Part print with two shaded views. Sizes in mm from the minimum x, y, z corner. A direction names the side the tool comes from. Give positions to 0.01 mm unless a question says otherwise; leave off trailing zeros. Loops run counter-clockwise (first coordinate to the right, second up) from the corner with the lowest first, then second, coordinate; pieces in that order, holes last. Notation, with made-up numbers: M 30.5,65 L 81.5,65 A29 ccw 81.5,87 Z; hole C 84.5,68.25 d1. An arc over 180 degrees is marked long. Answer in a Markdown table with one row per item.
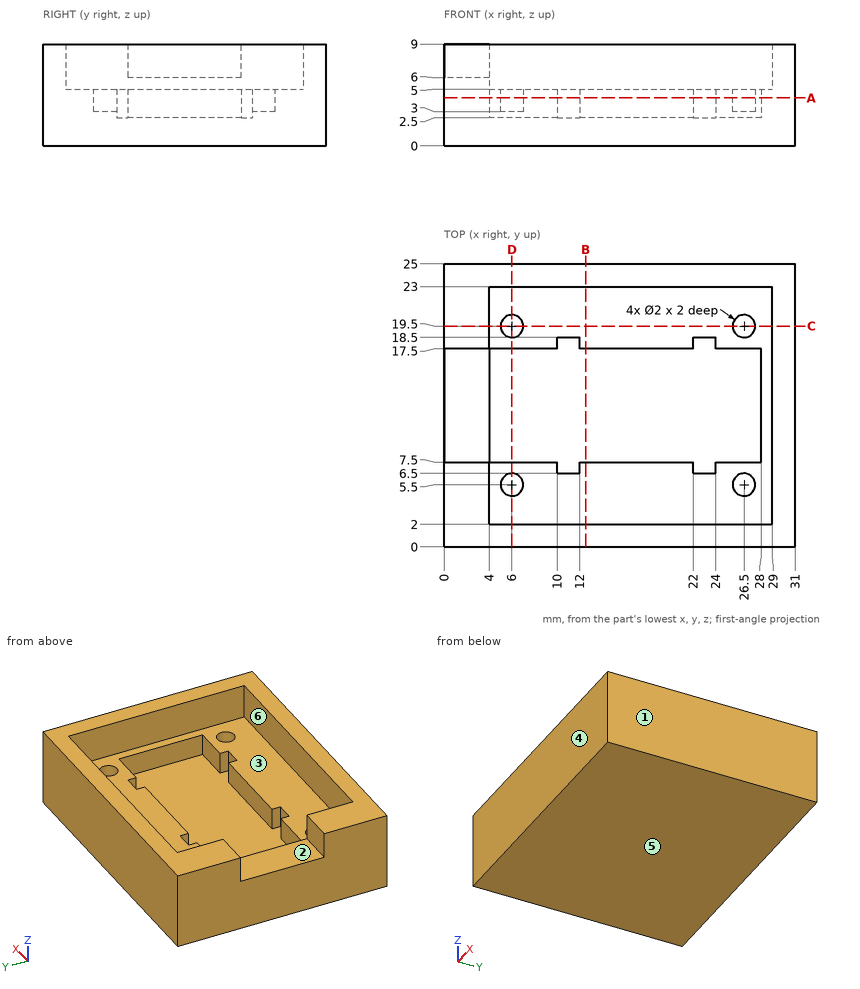
Q1. Saw through at D-D (x = 6). Give the cut face in (y, z), and give its area (3 significant figures).
Reported:
| item | result |
|---|---|
| outline | M 0,0 L 25,0 L 25,9 L 23,9 L 23,5 L 20.5,5 L 20.5,3 L 18.5,3 L 18.5,5 L 17.5,5 L 17.5,2.5 L 7.5,2.5 L 7.5,5 L 6.5,5 L 6.5,3 L 4.5,3 L 4.5,5 L 2,5 L 2,9 L 0,9 Z |
| area | 108 mm² |
Q2. Probe probe 1 along X at (y, z) = (19.5, 3.5); probe 2 along Y at (x, z) = (26.5, 4.4); probe 3 along Y at (x, z) = (12, 8.5). List the from-to ranges inside material, lowest first.
Reported:
| item | result |
|---|---|
| probe 1 | 0 to 5, 7 to 25.5, 27.5 to 31 |
| probe 2 | 0 to 4.5, 6.5 to 7.5, 17.5 to 18.5, 20.5 to 25 |
| probe 3 | 0 to 2, 23 to 25 |
Q3. Saw through at C-C (y = 19.5). Give the cut face in (x, z), and give its area (3 significant figures).
Reported:
| item | result |
|---|---|
| outline | M 0,0 L 31,0 L 31,9 L 29,9 L 29,5 L 27.5,5 L 27.5,3 L 25.5,3 L 25.5,5 L 7,5 L 7,3 L 5,3 L 5,5 L 4,5 L 4,9 L 0,9 Z |
| area | 171 mm² |
Q4. Mould opens along Y. For the marked faces 4, 5 and 6 say: released by +Y, released by -Y, zero draft, split by the parting line, or undercut.
Reported:
| item | result |
|---|---|
| face 4 | released by -Y |
| face 5 | zero draft |
| face 6 | undercut |
Q5. Saw through at B-B (x = 12.5). Give the cut face in (y, z), and give its area (3 significant figures).
Reported:
| item | result |
|---|---|
| outline | M 0,0 L 25,0 L 25,9 L 23,9 L 23,5 L 17.5,5 L 17.5,2.5 L 7.5,2.5 L 7.5,5 L 2,5 L 2,9 L 0,9 Z |
| area | 116 mm² |
Q6. Saw through at A-A (z = 4.25). Give the cut face in (x, y), and give its area (3 significant figures).
Reported:
| item | result |
|---|---|
| outline | M 0,0 L 31,0 L 31,25 L 0,25 Z; hole M 4,7.5 L 10,7.5 L 10,6.5 L 12,6.5 L 12,7.5 L 22,7.5 L 22,6.5 L 24,6.5 L 24,7.5 L 28,7.5 L 28,17.5 L 24,17.5 L 24,18.5 L 22,18.5 L 22,17.5 L 12,17.5 L 12,18.5 L 10,18.5 L 10,17.5 L 4,17.5 Z; hole C 6,5.5 d2; hole C 6,19.5 d2; hole C 26.5,5.5 d2; hole C 26.5,19.5 d2 |
| area | 514 mm² |
Q7. 3-axis set-ups, long thin cutter, end or side, ignore diameter. For the marked faces 1, 2 and 3: which of +Z, -Z, +X, -X, +Y, -Y reach the whole face in a straight line?
Reported:
| item | result |
|---|---|
| face 1 | +Z, -Z, +X, +Y, -Y |
| face 2 | +Z, -X |
| face 3 | +Z |
Q8. Drop flat-ended pins along their axis: pin 1 (1.6 mm diameter, centred on x = 26.5, y = 19.5, fed in from +Z); pin 2 (5 mm diameter, centred on x = 18, y = 7, fed in from +Z). Give the stop position or say it passes through.
Reported:
| item | result |
|---|---|
| pin 1 | z = 3 |
| pin 2 | z = 5 |
